For this review, take the finished solid that the model builds, in its own axes (mm). Face numbers are marked on the shaded views. Coordinates: 2 decimals unless noted, no trailing zeros. Order: outer loops, then holes, each group sorted by start corner. A loop starts at its lowest first (then second) coordinate and runs counter-clockwise, first axis right, second up.
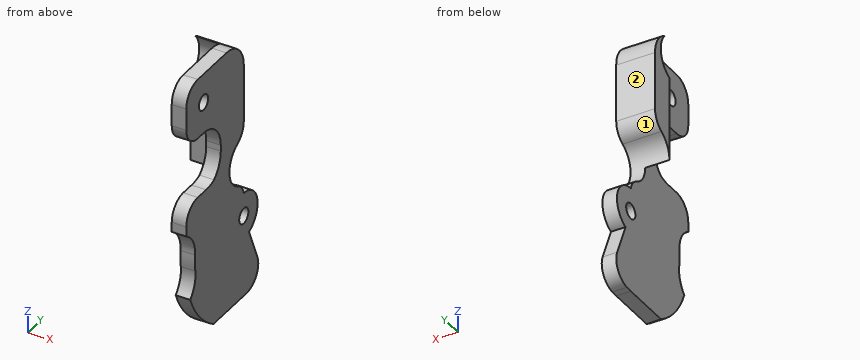
Autodesk Inventor part; units mm, degrees
ref_plane "YZ Plane" through (0, 0, 0) normal (1, 0, 0) x (0, 1, 0)
ref_plane "XZ Plane" through (0, 0, 0) normal (0, 1, 0) x (-1, 0, 0)
ref_plane "XY Plane" through (0, 0, 0) normal (0, 0, 1) x (1, 0, 0)
sketch "スケッチ1" plane through (0, 0, 0) normal (1, 0, 0) x (0, 1, 0)
  circle A0 centre (0, 0) radius 6 construction
  circle A1 centre (6, 0) radius 0.8
  line L0 (-14, 0) -> (14, 0)
  circle A2 centre (4.242641, 4.242641) radius 0.8
  circle A3 centre (0, 6) radius 0.8
  circle A4 centre (-4.242641, 4.242641) radius 0.8
  circle A5 centre (-6, 0) radius 0.8
  circle A6 centre (-4.242641, -4.242641) radius 0.8
  circle A7 centre (0, -6) radius 0.8
  circle A8 centre (4.242641, -4.242641) radius 0.8
  circle A9 centre (0, 0) radius 2.4
  line L1 (0, 0) -> (0, 6)
  line L2 (0, 0) -> (2.296101, -5.543277)
  circle A10 centre (0, 0) radius 10
  line L3 (2.296101, -5.543277) -> (3.826834, -9.238795)
  line L4 (0, -9.238795) -> (-10, -9.238795)
  line L5 (-10, -9.238795) -> (-10, 20)
  line L6 (-10, 20) -> (0, 20)
  line L7 (0, 20) -> (0, -9.238795)
  line L8 (0, -6) -> (4.242641, -4.242641) construction
  line L9 (0, -9.238795) -> (3.826834, -9.238795)
  circle A11 centre (0, 6) radius 2.5
  point P0 (0, 5.2)
  point P1 (0, 6.8)
  point P2 (-10, 0)
  point P3 (2.12132, -5.12132)
  point P4 (0, 2.4)
  point P5 (0.91844, -2.217311)
  point P6 (0, 8.5)
  point P7 (0, 10)
  point P8 (0, 3.5)
  point P9 (-3.826834, -9.238795)
  point P10 (0, -6.8)
  point P11 (0, -5.2)
  point P12 (0, -2.4)
  dimension "d1" = 12
  dimension "d2" = 1.6
  dimension "d5" = 360
  dimension "d7" = 4.8
  dimension "d8" = 4
  dimension "d21" = 5
  dimension "d23" = 20
sketch "スケッチ1 outline for 押し出し1" plane through (0, 0, 0) normal (1, 0, 0) x (0, 1, 0)
  arc A0 (0.91844, -2.217311) -> (0, 2.4) centre (0, 0) ccw
  line L0 (0, 2.4) -> (0, 3.5)
  arc A1 (0, 3.5) -> (0, 8.5) centre (0, 6) cw
  line L1 (0, 8.5) -> (0, 20)
  line L2 (0, 20) -> (-10, 20)
  line L3 (-10, 20) -> (-10, -9.238795)
  line L4 (-10, -9.238795) -> (3.826834, -9.238795)
  line L5 (3.826834, -9.238795) -> (0.91844, -2.217311)
extrude "押し出し1" add sketch "スケッチ1 outline for 押し出し1" along normal blind 1.5
sketch "スケッチ6" plane through (0, 0, 0) normal (-1, 0, 0) x (0, 0, 1)
  line L0 (12.746794, -7) -> (12.746794, -8)
  line L1 (17, -10) -> (14.746794, -10)
  line L2 (19, -8) -> (19, -3)
  arc A0 (19, -3) -> (16, 0) centre (16, -3) ccw
  line L3 (10.031129, 0) -> (16, 0)
  arc A1 (3.630208, 0.796296) -> (8.239516, -1.111111) centre (6, 0) ccw
  arc A2 (3.276042, 2.707407) -> (-3.926488, 1.626405) centre (0, 0) ccw
  line L4 (-5.713879, 2.366766) -> (-3.926488, 1.626405)
  arc A3 (-8.47286, 0.678702) -> (-8.5, 0) centre (0, 0) ccw
  line L5 (-8.5, 0) -> (-8.5, -5.267827)
  arc A4 (-8.5, -5.267827) -> (-3.6504, -9.309918) centre (0, 0) ccw
  arc A5 (-1.108696, -8.427384) -> (-3.6504, -9.309918) centre (-1.5, -11.401754) ccw
  arc A6 (-1.108696, -8.427384) -> (0.626747, -8.476862) centre (0, 0) ccw
  arc A7 (3.446028, -9.968696) -> (0.626747, -8.476862) centre (0.847952, -11.468696) ccw
  line L6 (3.446028, -9.968696) -> (3.464102, -10)
  line L7 (4.479657, -10) -> (3.464102, -10)
  line L8 (6.479657, -8) -> (6.479657, -6.559689)
  arc A8 (6.743932, -5.173913) -> (6.479657, -6.559689) centre (9.47607, -6.413035) ccw
  arc A9 (9.124144, -4) -> (6.743932, -5.173913) centre (9.124144, -7) ccw
  line L9 (9.124144, -4) -> (9.746794, -4)
  arc A10 (12.746794, -7) -> (9.746794, -4) centre (9.746794, -7) ccw
  circle A11 centre (17, -3.5) radius 0.8
  circle A12 centre (-6, 0) radius 0.8
  circle A13 centre (-4.242641, -4.242641) radius 0.8
  circle A14 centre (4.242641, -4.242641) radius 0.8
  circle A15 centre (0, -6) radius 0.8
  arc A16 (2.4, 0) -> (-2.217311, 0.91844) centre (0, 0) ccw
  line L10 (-9.238795, 3.826834) -> (-2.217311, 0.91844)
  line L11 (-9.238795, -10) -> (-9.238795, 3.826834)
  line L12 (20, -10) -> (-9.238795, -10)
  line L13 (20, 0) -> (20, -10)
  line L14 (8.5, 0) -> (20, 0)
  arc A17 (3.5, 0) -> (8.5, 0) centre (6, 0) ccw
  line L15 (2.4, 0) -> (3.5, 0)
  circle A18 centre (16, -7) radius 0.8
  circle A19 centre (0, 0) radius 0.8
  arc A20 (3.630208, 0.796296) -> (3.276042, 2.707407) centre (1.734375, 1.433333) ccw
  arc A21 (-5.713879, 2.366766) -> (-8.47286, 0.678702) centre (-6.479246, 0.519007) ccw
  arc A22 (4.479657, -10) -> (6.479657, -8) centre (4.479657, -8) ccw
  arc A23 (12.746794, -8) -> (14.746794, -10) centre (14.746794, -8) ccw
  arc A24 (17, -10) -> (19, -8) centre (17, -8) ccw
  arc A25 (10.031129, 0) -> (8.239516, -1.111111) centre (10.031129, -2) ccw
  point P0 (-7.852976, 3.252809)
  point P1 (6.479657, -10)
  point P2 (12.746794, -10)
  point P3 (16, 0)
  point P4 (19, -10)
  point P5 (-3.926488, 1.626405)
  point P6 (8.239516, -1.111111)
  point P7 (-3.926488, 1.626405)
  point P8 (16, 0)
sketch "スケッチ6 outline for 押し出し5" plane through (0, 0, 0) normal (-1, 0, 0) x (0, 0, 1)
  arc A0 (8.5, 0) -> (8.239516, -1.111111) centre (6, 0) cw
  line L0 (10.031129, 0) -> (8.5, 0)
  arc A1 (8.239516, -1.111111) -> (10.031129, 0) centre (10.031129, -2) cw
  line L1 (12.746794, -8) -> (12.746794, -7)
  arc A2 (14.746794, -10) -> (12.746794, -8) centre (14.746794, -8) cw
  line L2 (4.479657, -10) -> (14.746794, -10)
  arc A3 (6.479657, -8) -> (4.479657, -10) centre (4.479657, -8) cw
  line L3 (6.479657, -6.559689) -> (6.479657, -8)
  arc A4 (6.743932, -5.173913) -> (6.479657, -6.559689) centre (9.47607, -6.413035) ccw
  arc A5 (9.124144, -4) -> (6.743932, -5.173913) centre (9.124144, -7) ccw
  line L4 (9.746794, -4) -> (9.124144, -4)
  arc A6 (12.746794, -7) -> (9.746794, -4) centre (9.746794, -7) ccw
  line L5 (19, -3) -> (19, -8)
  arc A7 (16, 0) -> (19, -3) centre (16, -3) cw
  line L6 (20, 0) -> (16, 0)
  line L7 (20, -10) -> (20, 0)
  line L8 (17, -10) -> (20, -10)
  arc A8 (19, -8) -> (17, -10) centre (17, -8) cw
  arc A9 (-8.5, 0) -> (-8.47286, 0.678702) centre (0, 0) cw
  line L9 (-8.5, -5.267827) -> (-8.5, 0)
  arc A10 (-3.6504, -9.309918) -> (-8.5, -5.267827) centre (0, 0) cw
  arc A11 (-1.108696, -8.427384) -> (-3.6504, -9.309918) centre (-1.5, -11.401754) ccw
  arc A12 (0.626747, -8.476862) -> (-1.108696, -8.427384) centre (0, 0) cw
  arc A13 (3.446028, -9.968696) -> (0.626747, -8.476862) centre (0.847952, -11.468696) ccw
  line L10 (3.464102, -10) -> (3.446028, -9.968696)
  line L11 (-9.238795, -10) -> (3.464102, -10)
  line L12 (-9.238795, 3.826834) -> (-9.238795, -10)
  line L13 (-5.713879, 2.366766) -> (-9.238795, 3.826834)
  arc A14 (-8.47286, 0.678702) -> (-5.713879, 2.366766) centre (-6.479246, 0.519007) cw
extrude "押し出し5" cut sketch "スケッチ6 outline for 押し出し5" against normal through all
sketch "スケッチ7" plane through (0, 0, 0) normal (-1, 0, 0) x (0, 0, 1)
  line L0 (14.5, -3.5) -> (6.629791, -3.5)
  arc A0 (-7.852976, 3.252809) -> (-8.5, 0) centre (0, 0) ccw
  line L1 (-8.5, 0) -> (-8.5, -5.267827)
  arc A1 (-8.5, -5.267827) -> (-3.6504, -9.309918) centre (0, 0) ccw
  arc A2 (-1.108696, -8.427384) -> (-3.6504, -9.309918) centre (-1.5, -11.401754) ccw
  arc A3 (-1.108696, -8.427384) -> (0.626747, -8.476862) centre (0, 0) ccw
  arc A4 (3.446028, -9.968696) -> (0.626747, -8.476862) centre (0.847952, -11.468696) ccw
  line L2 (3.446028, -9.968696) -> (3.464102, -10)
  line L3 (6.479657, -10) -> (3.464102, -10)
  line L4 (6.479657, -10) -> (6.479657, -6.559689)
  arc A5 (6.743932, -5.173913) -> (6.479657, -6.559689) centre (9.47607, -6.413035) ccw
  arc A6 (9.124144, -4) -> (6.743932, -5.173913) centre (9.124144, -7) ccw
  line L5 (9.124144, -4) -> (9.746794, -4)
  arc A7 (12.746794, -7) -> (9.746794, -4) centre (9.746794, -7) ccw
  line L6 (12.746794, -7) -> (12.746794, -10)
  line L7 (19, -10) -> (12.746794, -10)
  line L8 (19, -10) -> (19, -3)
  arc A8 (19, -3) -> (16, 0) centre (16, -3) ccw
  line L9 (8.5, 0) -> (16, 0)
  arc A9 (3.5, 0) -> (8.5, 0) centre (6, 0) ccw
  line L10 (2.4, 0) -> (3.5, 0)
  arc A10 (2.4, 0) -> (-2.217311, 0.91844) centre (0, 0) ccw
  line L11 (-7.852976, 3.252809) -> (-2.217311, 0.91844)
  circle A11 centre (17, -3.5) radius 0.8
  circle A12 centre (17, -3.5) radius 2.5
  line L12 (6.629791, -3.5) -> (0, -3.5)
  circle A13 centre (0, 0) radius 3.5
  line L13 (3.5, 0) -> (3.5, -3.5)
  line L14 (0, -3.5) -> (14.708712, -3.5)
  line L15 (14.708712, -3.5) -> (14.708712, -2.5)
  line L16 (14.708712, -2.5) -> (0, -2.5)
  line L17 (0, -2.5) -> (0, -3.5)
  point P0 (18.677033, -1.645934)
  point P1 (6, -2.5)
  dimension "d31" = 5
  dimension "d34" = 1
sketch "スケッチ7 outline for 押し出し6" plane through (0, 0, 0) normal (-1, 0, 0) x (0, 0, 1)
  line L0 (16, 0) -> (8.5, 0)
  arc A0 (18.677033, -1.645934) -> (16, 0) centre (16, -3) ccw
  arc A1 (14.708712, -2.5) -> (18.677033, -1.645934) centre (17, -3.5) cw
  line L1 (6, -2.5) -> (14.708712, -2.5)
  arc A2 (8.5, 0) -> (6, -2.5) centre (6, 0) cw
extrude "押し出し6" add sketch "スケッチ7 outline for 押し出し6" along normal blind 2.5
sketch "スケッチ8" plane through (1.5, 0, 0) normal (1, 0, 0) x (0, 0, -1)
  circle A0 centre (-16, -7) radius 0.8
  line L0 (-17, -10) -> (-14.746794, -10)
  line L1 (-19, -3) -> (-19, -8)
  circle A1 centre (0, 0) radius 0.8
  point P0 (-19, -10)
  point P1 (-12.746794, -10)
  dimension "d35" = 1.6
  dimension "d36" = 3
  dimension "d37" = 3
  dimension "d40" = 1.6
sketch "スケッチ8 outline for 押し出し7" plane through (1.5, 0, 0) normal (1, 0, 0) x (0, 0, -1)
  circle A0 centre (-16, -7) radius 0.8
  circle A1 centre (0, 0) radius 0.8
extrude "押し出し7" cut sketch "スケッチ8 outline for 押し出し7" against normal through all
fillet "フィレット1" radius 2 2 edges at (0.75, 0, 3.5) (-1.25, 0, 8.5)
properties part number "toe_springjoint_cover_under_left"
1. Take a section at C-C, the plane y = 1.75. Give the boundary of the cut face in (x, z), plus the area to 3 significant figures.
Answer below:
outline: (0, -8.06) - (1.5, -8.06) - (1.5, -4.22) - (0, -4.22) - close; (0, -1.64) - (1.5, -1.64) - (1.5, 1.64) - (0, 1.64) - close
area: 10.7 mm2
2. Take a section at B-B, the plane y = -8.75. Give the boundary of the cut face in (x, z), plus the area to 3 significant figures.
Answer below:
outline: (0, -4.84) - (1.5, -4.84) - (1.5, -2.9) - (0, -2.9) - close; (0, 2.12) - (1.5, 2.12) - (1.5, 6.33) - (0, 6.33) - close; (0, 12.89) - (1.5, 12.89) - (1.5, 18.85) - (0, 18.85) - close
area: 18.2 mm2
3. To check wall thickness, follow L1, parallel to Y at x = 0.9, z = 0; L2, parallel to Y at x = 0.55, z = 16; L3, parallel to X at y = -4.5, z = -5. State the ranges of each line that lie inside material, in increasing order.
Answer below:
L1: y = -8.5 to -0.8, 0.8 to 2.4
L2: y = -10 to -7.8, -6.2 to 0
L3: x = 0 to 1.5
4. The part is to be moulded in two halves that separate along Z. For the marked faces 1 and 2, say which applies: +Z half, -Z half, draft (parallel to the pull), parting line (faces both ways), or undercut.
Answer below:
face 1: undercut
face 2: draft
5. Take a section at D-D, the plane z = 13.25. Give the boundary of the cut face in (x, y).
Answer below:
outline: (-2.5, -2.5) - (0, -2.5) - (0, -9.33) - (1.5, -9.33) - (1.5, 0) - (-2.5, 0) - close
6. Clearance check with flat-ended pins moving along their axes: pin 1 Ø5 at (y, z) = (0, 8) entering from +X; pin 2 Ø0.5 at (x, y) = (0.5, -7.5) entering from -Z; pin 3 Ø0.5 at (x, z) = (1, 9.5) entering from -Y; pin 4 Ø0.8 at (x, z) = (-0.5, 12.5) entering from -Y. State where each tip first meets the part, or that it passes through.
Answer below:
pin 1: stops at x = 1.5
pin 2: stops at z = -6.89
pin 3: stops at y = -4
pin 4: stops at y = -2.5
7. Take a section at A-A, the plane z = 0. Give the boundary of the cut face in (x, y).
Answer below:
outline: (0, -8.5) - (1.5, -8.5) - (1.5, -0.8) - (0, -0.8) - close; (0, 0.8) - (1.5, 0.8) - (1.5, 2.4) - (0, 2.4) - close
